Design review of the part built by this model. Coordinates are the model's own, in mm. A direction names the side the tool comes from. Round coordinates to 2 decimals unless told otherwise and drop trailing zeros. Loops run counter-clockwise (first coordinate to the right, second up) from the corner with the lowest first, then second, coordinate; pieces in that order, holes last. Notation, with made-up numbers: (69.25, 55.5) - (121.25, 55.5) arc R16 cw to (121.25, 61.5) - close; hole circle Ø4 at (-36.75, -27). An arc over 180 degrees is marked (long way). Return JSON: item names as keys, results as strings. Group by question number.
from build123d import *

# Parameters (mm, degrees)
BOSS_EXTRUDE1_DEPTH = 28.575
SKETCH3_R           = 15.875
CUT_EXTRUDE1_DEPTH  = 12.7
SKETCH4_R           = 12.7
CUT_EXTRUDE2_DEPTH  = 12.7


with BuildPart() as part:
    # Sketch2 → Boss-Extrude1 (new, symmetric)
    with BuildSketch(Plane.XY):
        Polygon((0, 0), (69.85, 0), (69.85, 25.4), (130.175, 25.4), (130.175, 38.1), (57.15, 38.1), (57.15, 12.7), (12.7, 12.7), (12.7, 38.1), (0, 38.1), align=None)
    extrude(amount=BOSS_EXTRUDE1_DEPTH, both=True)

    # Sketch3 → Cut-Extrude1 (cut)
    with BuildSketch(Plane(origin=(0, 12.7, 0), x_dir=(1, 0, 0), z_dir=(0, 1, 0))):
        with Locations(Location((34.925, 0, 0), (0, 0, 180))):
            Circle(SKETCH3_R)
    extrude(amount=-CUT_EXTRUDE1_DEPTH, mode=Mode.SUBTRACT)

    # Sketch4 → Cut-Extrude2 (cut)
    with BuildSketch(Plane(origin=(0, 38.1, 0), x_dir=(1, 0, 0), z_dir=(0, 1, 0))):
        with Locations(Location((101.6, 0, 0), (0, 0, 180))):
            Circle(SKETCH4_R)
        with BuildLine():
            Line((130.175, 28.575), (102.896747677, 28.575))
            ThreePointArc((102.896747677, 28.575), (121.826371147, 20.226371147), (130.175, 1.296747677))
            Line((130.175, 1.296747677), (130.175, 28.575))
        make_face()
        with BuildLine():
            Line((130.175, -28.575), (130.175, -1.296747677))
            ThreePointArc((130.175, -1.296747677), (121.826371147, -20.226371147), (102.896747677, -28.575))
            Line((102.896747677, -28.575), (130.175, -28.575))
        make_face()
    extrude(amount=-CUT_EXTRUDE2_DEPTH, mode=Mode.SUBTRACT)


solid = part.part
Q1. For line 1 (Z direction, x = 101, y = 34) (3 decimals); line 2 (X direction, y = 34, z = -9.5); line 3 (X direction, y = 17, z = 12), list the stretches that pass through material, from the lowest coordinate up.
Q2. Add section D-D, the plane y = 14.5. State the section outline as (x, z) points (3 decimals).
Q3. Tool access review of faces 4 (the cylindrical face through (121.62, 31.84, -20.43)), 5 (the flat face through (12.7, 25, 0)): name each direction out of +Z, -Z, +X, -X, +Y, -Y from which nothing blocks a thin tool from reaching the whole face with its end or side.
Q4. Add section B-B, the plane y = 35. State the section outline as (x, z) points (3 decimals).
Q5. Add section C-C, the plane x = 101.6. State the section outline as (y, z) points (3 decimals), plus the area to 3 significant figures.
Q6. Insertion check: pin 1 Ø5 at (y, z) = (6, 18.5) entering from +X; pin 2 Ø15 at (x, z) = (101.6, 0) entering from +Y; pin 3 Ø6 at (x, z) = (52.5, -2.5) entering from +Y. Each pin has a flat end and moves straight along its axis. Give the tip position at first contact, or say it passes through.
Q7. Add section A-A, the plane z = 0. State the section outline as (x, y) points (3 decimals), plus the area to 3 significant figures.
Q8. Draft analysis for pull direction X (two halves, no side actions). For faces 1 (the flat face through (86, 25.4, 0)), 2 (the flat face through (69.85, 13, 0)), 3 (the flat face through (45, 12.7, 13)), state which applies: pulls with the +X half, pulls with the -X half, needs draft (parallel to the pull), parting line crosses it, or undercut.
Evaluation:
{
 "1": {"line 1": "-28.575 to -12.686, 12.686 to 28.575", "line 2": "0 to 12.7, 57.15 to 93.17, 110.03 to 128.58", "line 3": "0 to 12.7, 57.15 to 69.85"},
 "2": {"outline": "(0, -28.575) - (12.7, -28.575) - (12.7, 28.575) - (0, 28.575) - close; (57.15, -28.575) - (69.85, -28.575) - (69.85, 28.575) - (57.15, 28.575) - close"},
 "3": {"face 4": "-Z, +X, +Y, -Y", "face 5": "+Z, -Z, +Y"},
 "4": {"outline": "(0, -28.575) - (12.7, -28.575) - (12.7, 28.575) - (0, 28.575) - close; (57.15, -28.575) - (102.897, -28.575) arc R28.604 ccw to (130.175, -1.297) - (130.175, 1.297) arc R28.604 ccw to (102.897, 28.575) - (57.15, 28.575) - close; hole circle Ø25.4 at (101.6, 0)"},
 "5": {"outline": "(25.4, -28.575) - (38.1, -28.575) - (38.1, -12.7) - (25.4, -12.7) - close; (25.4, 12.7) - (38.1, 12.7) - (38.1, 28.575) - (25.4, 28.575) - close", "area": "403 mm²"},
 "6": {"pin 1": "x = 69.85", "pin 2": "through", "pin 3": "y = 12.7"},
 "7": {"outline": "(0, 0) - (19.05, 0) - (19.05, 12.7) - (12.7, 12.7) - (12.7, 38.1) - (0, 38.1) - close; (50.8, 0) - (69.85, 0) - (69.85, 25.4) - (88.9, 25.4) - (88.9, 38.1) - (57.15, 38.1) - (57.15, 12.7) - (50.8, 12.7) - close; (114.3, 25.4) - (130.175, 25.4) - (130.175, 38.1) - (114.3, 38.1) - close", "area": "1,570 mm²"},
 "8": {"face 1": "needs draft", "face 2": "pulls with the +X half", "face 3": "undercut"}
}
